Design review of the part built by this model. Coordinates are the model's own, in mm. Face numbers are marked on the shaded views. A direction names the side the tool comes from. Round coordinates to 2 decimals unless told otherwise and drop trailing zeros. Loops run counter-clockwise (first coordinate to the right, second up) from the corner with the lowest first, then second, coordinate; pieces in that order, holes last. Notation, with made-up numbers: (-2.5, -21) -> (19.5, -21) arc R23 cw to (19.5, 14) -> close; hole circle Ø9 at (71, 26). An arc over 180 degrees is marked (long way). Write each question's results on one line, items separated by ' | '. Start each with the question number.
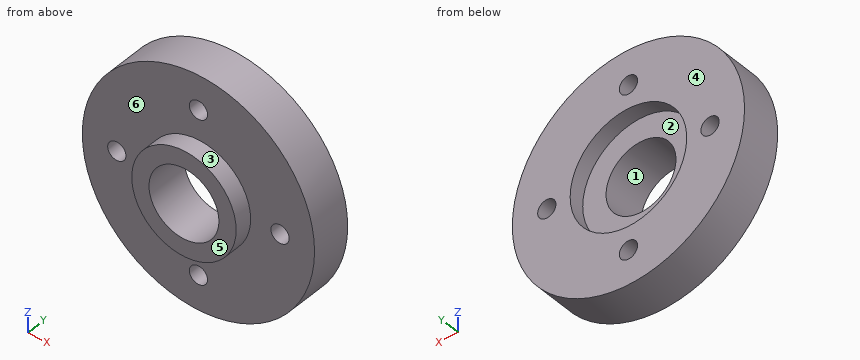
Autodesk Inventor part; units mm, degrees
ref_plane "YZ Plane" through (0, 0, 0) normal (1, 0, 0) x (0, 1, 0)
ref_plane "XZ Plane" through (0, 0, 0) normal (0, 1, 0) x (-1, 0, 0)
ref_plane "XY Plane" through (0, 0, 0) normal (0, 0, 1) x (1, 0, 0)
sketch "스케치1" plane through (0, 0, 0) normal (0, 0, 1) x (1, 0, 0)
  line L0 (0, 6.4532) -> (0, -6.4532)
  line L1 (3, -3.68) -> (3, 0)
  line L2 (3, 0) -> (5, 0)
  line L3 (5, 0) -> (5, 1.32)
  line L4 (5, 1.32) -> (9.96, 1.32)
  line L5 (9.96, 1.32) -> (9.96, -2.16)
  line L6 (9.96, -2.16) -> (4.48, -2.16)
  line L7 (4.48, -2.16) -> (4.48, -3.68)
  line L8 (4.48, -3.68) -> (3, -3.68)
  point P0 (0, 0)
  point P1 (0, 0)
  dimension "d22" = 6
  dimension "d23" = 8.96
  dimension "d24" = 10
  dimension "d25" = 19.92
  dimension "d26" = 1.32
  dimension "d27" = 5
  dimension "d28" = 3.48
revolve "회전1" add sketch "스케치1" angle 360 about axis through (0, 6.4532, 0) along (0, -1, 0)
sketch "Sketch3" plane through (0, 1.32, 0) normal (0, 1, 0) x (1, 0, 0)
  point P0 (0, 0)
  point P1 (7, 0)
  point P2 (0, 7)
  point P3 (-7, 0)
  point P4 (0, -7)
  dimension "d29" = 7
  dimension "d32" = 360
hole "Hole2" at (7, 1.32, 0) at (0, 1.32, -7) at (-7, 1.32, 0) at (0, 1.32, 7) direction (0, -1, 0) diameter 1.567 end through all
properties part number "Bottom Horn" material "Aluminum 6061-AHC"
1) Take a section at B-B (z = 0). Write out the cut boundary in (x, y).
2) Take a section at D-D (z = 7). Write out the cut boundary in (x, y), plus the area to 3 significant figures.
3) For the marked faces 5 and 6, list the 3-axis set-ups (+Z, -Z, +X, -X, +Y, -Y) from which the entire face can be reached by the end or side of a thin tool; tool diameter is ignored.
4) To check wall thickness, follow line 1 (Z direction, x = 0, y = -1.4); line 2 (Z direction, x = 0, y = 1); line 3 (X direction, y = 1, z = 0.5). State the ranges of each line that lie inside material, in increasing order. Write a range as from..to.
5) Take a section at A-A (x = 0). Write out the cut boundary in (y, z).
6) Take a section at C-C (y = -1.55). Write out the cut boundary in (x, z).
7) Insertion check: pin 1 (0.9 mm diameter, centred on x = 0, z = -7, fed in from -Y); pin 2 (3 mm diameter, centred on y = 0, z = -6, fed in from +X); pin 3 (6 mm diameter, centred on x = -7.5, z = 4.5, fed in from -Y); pin 4 (2 mm diameter, centred on y = -2.5, z = 4, fed in from -X). Each pin has a flat end and moves straight along its axis. Give the tip position at first contact, or say it passes through.
8) The part is to be moulded in two halves that separate along Z. For the marked faces 1, 2, 3 and 4, say which applies: +Z half, -Z half, draft (parallel to the pull), parting line (faces both ways), or undercut.
Geometry check:
1) outline: (-9.96, -2.16) -> (-7.78, -2.16) -> (-7.78, 1.32) -> (-9.96, 1.32) -> close; (-6.22, -2.16) -> (-4.48, -2.16) -> (-4.48, -3.68) -> (-3, -3.68) -> (-3, 0) -> (-5, 0) -> (-5, 1.32) -> (-6.22, 1.32) -> close; (3, -3.68) -> (4.48, -3.68) -> (4.48, -2.16) -> (6.22, -2.16) -> (6.22, 1.32) -> (5, 1.32) -> (5, 0) -> (3, 0) -> close; (7.78, -2.16) -> (9.96, -2.16) -> (9.96, 1.32) -> (7.78, 1.32) -> close
2) outline: (-7.09, -2.16) -> (-0.78, -2.16) -> (-0.78, 1.32) -> (-7.09, 1.32) -> close; (0.78, -2.16) -> (7.09, -2.16) -> (7.09, 1.32) -> (0.78, 1.32) -> close | area: 43.9 mm^2
3) face 5: +Z, -Z, +X, -X, -Y | face 6: -Y
4) line 1: z = -9.96..-7.78, -6.22..-3, 3..6.22, 7.78..9.96 | line 2: z = -9.96..-7.78, -6.22..-5, 5..6.22, 7.78..9.96 | line 3: x = -9.95..-7.6, -6.4..-4.97, 4.97..6.4, 7.6..9.95
5) outline: (-3.68, -4.48) -> (-2.16, -4.48) -> (-2.16, -6.22) -> (1.32, -6.22) -> (1.32, -5) -> (0, -5) -> (0, -3) -> (-3.68, -3) -> close; (-3.68, 3) -> (0, 3) -> (0, 5) -> (1.32, 5) -> (1.32, 6.22) -> (-2.16, 6.22) -> (-2.16, 4.48) -> (-3.68, 4.48) -> close; (-2.16, -9.96) -> (1.32, -9.96) -> (1.32, -7.78) -> (-2.16, -7.78) -> close; (-2.16, 7.78) -> (1.32, 7.78) -> (1.32, 9.96) -> (-2.16, 9.96) -> close
6) outline: circle Ø19.92 at (0, 0); hole circle Ø1.57 at (-7, 0); hole circle Ø6 at (0, 0); hole circle Ø1.57 at (0, -7); hole circle Ø1.57 at (0, 7); hole circle Ø1.57 at (7, 0)
7) pin 1: passes through | pin 2: stops at x = 8.89 | pin 3: stops at y = -2.16 | pin 4: stops at x = -9.48
8) face 1: undercut | face 2: undercut | face 3: parting line | face 4: draft
